Input: part model. Units: mm. Frame: model coordinates. Give positions to 0.01 mm unless a question says otherwise; leave off trailing zeros. Loops run counter-clockwise (first coordinate to the right, second up) from the corner with the lowest first, then second, coordinate; pieces in that order, holes last.
from build123d import *

# Parameters (mm, degrees)
BOX005_W     = 25
BOX005_H     = 10
BOX005_DEPTH = 10
BOX004_W     = 25
BOX004_H     = 10
BOX004_DEPTH = 10
BOX001_W     = 297
BOX001_H     = 10
BOX001_DEPTH = 2


with BuildPart() as cube005:
    # Box005 → Box005 (new body)
    with BuildSketch(Plane(origin=(272, 0, 0), x_dir=(1, 0, 0), z_dir=(0, 0, 1))):
        with Locations((12.5, 5)):
            Rectangle(BOX005_W, BOX005_H)
    extrude(amount=BOX005_DEPTH)


with BuildPart() as cube004:
    # Box004 → Box004 (new body)
    with BuildSketch(Plane.XY):
        with Locations((12.5, 5)):
            Rectangle(BOX004_W, BOX004_H)
    extrude(amount=BOX004_DEPTH)


with BuildPart() as cone004:
    # Cone004 → Cone004 (revolve)
    with BuildSketch(Plane(origin=(31.5, 5, 0), x_dir=(1, 0, 0), z_dir=(0, -1, 0))):
        Polygon((0, 0), (0.2, 0), (1.5, 2), (0, 2), align=None)
    revolve(axis=Axis((31.5, 5, 0), (0, 0, 1)))


with BuildPart() as cone005:
    # Cone005 → Cone005 (revolve)
    with BuildSketch(Plane(origin=(114.5, 5, 0), x_dir=(1, 0, 0), z_dir=(0, -1, 0))):
        Polygon((0, 0), (0.2, 0), (1.5, 2), (0, 2), align=None)
    revolve(axis=Axis((114.5, 5, 0), (0, 0, 1)))


with BuildPart() as cone006:
    # Cone006 → Cone006 (revolve)
    with BuildSketch(Plane(origin=(182.5, 5, 0), x_dir=(1, 0, 0), z_dir=(0, -1, 0))):
        Polygon((0, 0), (0.2, 0), (1.5, 2), (0, 2), align=None)
    revolve(axis=Axis((182.5, 5, 0), (0, 0, 1)))


with BuildPart() as cone007:
    # Cone007 → Cone007 (revolve)
    with BuildSketch(Plane(origin=(265.5, 5, 0), x_dir=(1, 0, 0), z_dir=(0, -1, 0))):
        Polygon((0, 0), (0.2, 0), (1.5, 2), (0, 2), align=None)
    revolve(axis=Axis((265.5, 5, 0), (0, 0, 1)))


with BuildPart() as obj1:
    # Box001 → Box001 (new body)
    with BuildSketch(Plane.XY.offset(2)):
        with Locations((148.5, 5)):
            Rectangle(BOX001_W, BOX001_H)
    extrude(amount=BOX001_DEPTH)

    # Fusion: union Cone007
    add(cone007.part)

    # Fusion001: union Cone006
    add(cone006.part)

    # Fusion002: union Cone005
    add(cone005.part)

    # Fusion003: union Cone004
    add(cone004.part)

    # Cut005: cut Cube004
    add(cube004.part, mode=Mode.SUBTRACT)

    # Cut006: cut Cube005
    add(cube005.part, mode=Mode.SUBTRACT)


solid = obj1.part
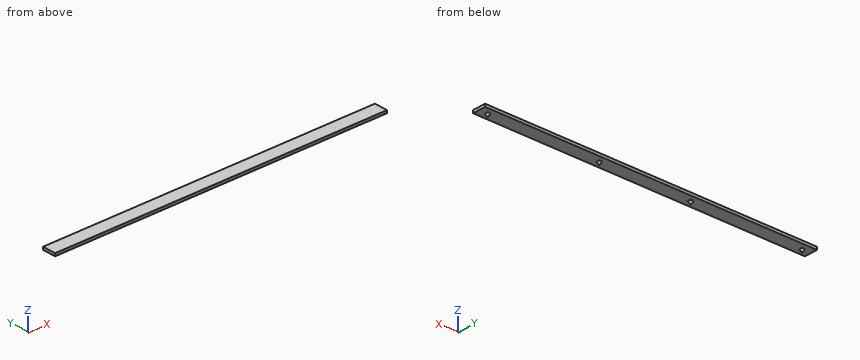
(1) Cut plane B-B (y = 1.75). Return the cut outline in (x, z).
Values follow:
outline: (25, 2) - (272, 2) - (272, 4) - (25, 4) - close
(2) Cut plane C-C (x = 247.5). Return the cut outline in (y, z), and give its area (3 significant figures).
Values follow:
outline: (0, 2) - (10, 2) - (10, 4) - (0, 4) - close
area: 20.0 mm2
(3) Cut plane A-A (z = 1.2). Return the cut outline in (x, y).
Values follow:
outline: circle Ø1.96 at (31.5, 5); circle Ø1.96 at (114.5, 5); circle Ø1.96 at (182.5, 5); circle Ø1.96 at (265.5, 5)
(4) Ray query, probe 1 along Z at (x, y) = (261, 4); probe 2 along X at (y, z) = (4.5, 1.25). Return the intervals inside material, ascending.
Values follow:
probe 1: z = 2 to 4
probe 2: x = 30.62 to 32.38, 113.62 to 115.38, 181.62 to 183.38, 264.62 to 266.38
(5) Pin query (flat end, axial travel): pin 1 Ø2 at (x, z) = (201, 3.5) entering from -Y. Return the tip coordinate at first contact, or that it passes through.
Values follow:
pin 1: stops at y = 0
